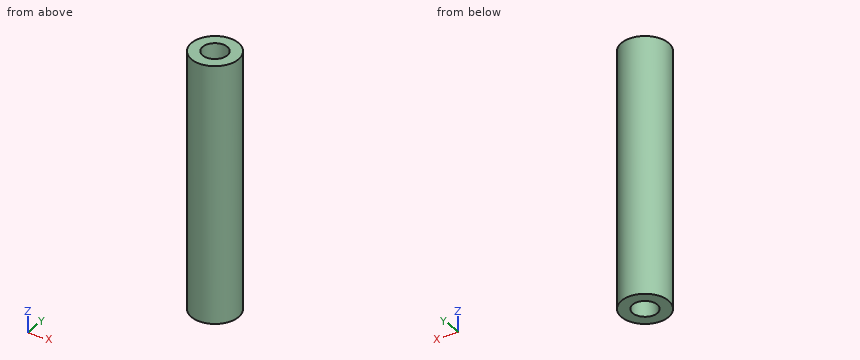
```python
from build123d import *

# Parameters (mm, degrees)
SKETCH1_R           = 6
BOSS_EXTRUDE1_DEPTH = 65.5
SKETCH2_R           = 1
CUT_EXTRUDE1_DEPTH  = 66.5
SKETCH3_R           = 3.14325
CUT_EXTRUDE2_DEPTH  = 9.0297
CUT_EXTRUDE2_TAPER  = 2.328
SKETCH4_R           = 3.14325
CUT_EXTRUDE3_DEPTH  = 9.0297
CUT_EXTRUDE3_TAPER  = 2.328


with BuildPart() as part:
    # Sketch1 → Boss-Extrude1 (new body)
    with BuildSketch(Plane.XY):
        Circle(SKETCH1_R)
    extrude(amount=BOSS_EXTRUDE1_DEPTH)

    # Sketch2 → Cut-Extrude1 (cut, through all)
    with BuildSketch(Plane.XY):
        Circle(SKETCH2_R)
    extrude(amount=CUT_EXTRUDE1_DEPTH, mode=Mode.SUBTRACT)

    # Sketch3 → Cut-Extrude2 (cut)
    with BuildSketch(Plane.XY):
        Circle(SKETCH3_R)
    extrude(amount=CUT_EXTRUDE2_DEPTH, taper=CUT_EXTRUDE2_TAPER, mode=Mode.SUBTRACT)

    # Sketch4 → Cut-Extrude3 (cut)
    with BuildSketch(Plane.XY.offset(65.5)):
        Circle(SKETCH4_R)
    extrude(amount=-CUT_EXTRUDE3_DEPTH, taper=CUT_EXTRUDE3_TAPER, mode=Mode.SUBTRACT)


solid = part.part
```
Work out the finished part from the listing and answer in its coordinate system (mm). Round coordinates to 2 decimals unless told otherwise and drop trailing zeros. Loops run counter-clockwise (first coordinate to the right, second up) from the corner with the lowest first, then second, coordinate; pieces in that order, holes last.
(1) Find the intervals of material crossed by L1, parallel to Y at x = 0, z = 24; L2, parallel to X at y = -0.25, z = 30; L3, parallel to Z at x = 1, y = -0.75, in increasing order.
Computed values:
L1: y = -6 to -1, 1 to 6
L2: x = -5.99 to -0.97, 0.97 to 5.99
L3: z = 9.03 to 56.47
(2) The part is cut by section A-A, the plane x = 0. Give the vertices of the cut face in (y, z), and give its area (3 significant figures).
Computed values:
outline: (-6, 0) - (-3.14, 0) - (-2.78, 9.03) - (-1, 9.03) - (-1, 56.47) - (-2.78, 56.47) - (-3.14, 65.5) - (-6, 65.5) - close; (1, 9.03) - (2.78, 9.03) - (3.14, 0) - (6, 0) - (6, 65.5) - (3.14, 65.5) - (2.78, 56.47) - (1, 56.47) - close
area: 584 mm2
(3) The part is cut by section C-C, the plane y = 4.75. Give the vertices of the cut face in (x, z).
Computed values:
outline: (-3.67, 0) - (3.67, 0) - (3.67, 65.5) - (-3.67, 65.5) - close
(4) The part is cut by section B-B, the plane z = 39.5. Give the vertices of the cut face in (x, y).
Computed values:
outline: circle Ø12 at (0, 0); hole circle Ø2 at (0, 0)
(5) The part is cut by section D-D, the plane x = 4.25. Give the vertices of the cut face in (y, z), and give its area (3 significant figures).
Computed values:
outline: (-4.24, 0) - (4.24, 0) - (4.24, 65.5) - (-4.24, 65.5) - close
area: 555 mm2
(6) Each of these flat-tipped pins is pushed along its axis until it touches: P1, Ø1, axis at y = -2, z = 29, coming from the -X side; P2, Ø1, axis at x = 2.5, z = 54, coming from the +Y side; P3, Ø1, axis at x = 3.5, z = 10, coming from the +Y side. Where does it stop, or does it pass through?
Computed values:
P1: stops at x = -5.81
P2: stops at y = 5.66
P3: stops at y = 5.2
